Part model, mm, in its own coordinate system. Face numbers are marked on the shaded views. Give positions to 0.01 mm unless a question says otherwise; leave off trailing zeros. Write each loop counter-clockwise with the first axis right and the second up, starting at its lowest first coordinate (ties: lowest second). Pieces come first, ordered by that corner, then holes. Notation, with made-up numbers: (8.25, 12) - (35.25, 12) arc R32 cw to (35.25, 45) - close; hole circle Ø7 at (24, 62). An arc over 180 degrees is marked (long way). Answer as a JSON object with one key per item and string values. Group by question number.
```python
from build123d import *

# Parameters (mm, degrees)
ESQUISSE2_W             = 1
ESQUISSE2_H             = 6
ENL_V_MAT_EXTRU_1_DEPTH = 0.5


with BuildPart() as part:
    # Esquisse1 → Révolution1 (revolve)
    with BuildSketch(Plane.XY):
        Polygon((0, 0), (3, 0), (3, 1), (1.5, 1), (1.5, 10), (0, 10), align=None)
    revolve(axis=Axis((0, 0, 0), (0, 1, 0)))

    # Esquisse2 → Enlèv. mat.-Extru.1 (cut)
    with BuildSketch(Plane.XZ):
        Rectangle(ESQUISSE2_W, ESQUISSE2_H)
    extrude(amount=-ENL_V_MAT_EXTRU_1_DEPTH, mode=Mode.SUBTRACT)


solid = part.part
```
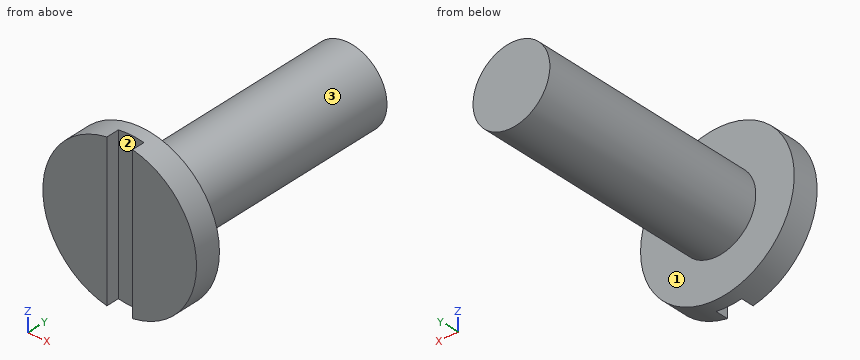
1) Saw through at D-D (x = -1.3). List the corners of the cut face in (y, z).
2) Two-plate mould, pull along X, no slides. Class the marked faces 1, 2 and 3: +X half, -X half, draft (parallel to the pull), parting line (faces both ways), or undercut.
3) Saw through at C-C (y = 5.25). List the corners of the cut face in (x, z).
4) Drill centre lines: line 1 along X through (y, z) = (9.5, 0); line 2 along Y through (x, z) = (-0.05, -1); line 3 along Y through (x, z) = (-0.7, 1.5). Where is each one in solid material? Low to high. Write a range as from..to.
5) Saw through at B-B (x = 0). List the corners of the cut face in (y, z).
6) Saw through at A-A (z = 0). List the corners of the cut face in (x, y), and give its area (3 significant figures).
7) Drop flat-ended pins along their axis: P1, Ø3, axis at x = -2, y = 1.5, coming from the +Z side; P2, Ø2, axis at x = -1, y = 6, coming from the -Z side; P3, Ø3, axis at x = -2.5, y = 5, coming from the +Z side. Give the stop position or say it passes through.
Checks:
{
 "1": {"outline": "(0, -2.7) - (1, -2.7) - (1, -0.75) - (10, -0.75) - (10, 0.75) - (1, 0.75) - (1, 2.7) - (0, 2.7) - close"},
 "2": {"face 1": "draft", "face 2": "undercut", "face 3": "parting line"},
 "3": {"outline": "circle Ø3 at (0, 0)"},
 "4": {"line 1": "-1.5..1.5", "line 2": "0.5..10", "line 3": "0..1"},
 "5": {"outline": "(0.5, -3) - (1, -3) - (1, -1.5) - (10, -1.5) - (10, 1.5) - (1, 1.5) - (1, 3) - (0.5, 3) - close"},
 "6": {"outline": "(-3, 0) - (-0.5, 0) - (-0.5, 0.5) - (0.5, 0.5) - (0.5, 0) - (3, 0) - (3, 1) - (1.5, 1) - (1.5, 10) - (-1.5, 10) - (-1.5, 1) - (-3, 1) - close", "area": "32.5 mm2"},
 "7": {"P1": "z = 2.94", "P2": "z = -1.5", "P3": "z = 1.12"}
}
